Input: part model. Units: mm. Frame: model coordinates. Round coordinates to 2 decimals unless told otherwise and drop trailing zeros. Loops run counter-clockwise (first coordinate to the right, second up) from the corner with the lowest first, then second, coordinate; pieces in that order, holes last. Notation, with made-up numbers: (27, 58.5) -> (71, 58.5) arc R23 ccw to (71, 70.5) -> close; hole circle Ø9 at (87, 70). An arc over 180 degrees is marked (long way). Answer as a JSON object with one key per item and string values. Group by question number.
Item 1: Section query A-A on x = -4. Return loops of the section in (y, z).
Item 2: Section query B-B on x = 132.5. Return loops of the section in (y, z), and give its area (3 significant figures).
Item 3: Material intervals for line 1 (Z direction, x = -11.5, y = 0); line 2 (Y direction, x = -7, z = 3); line 3 (Z direction, x = -16.5, y = -3.5), sorted ascending. Write a range as [from, to].
Item 4: Draft query along Z for faces 1 (the cylindrical face through (-14.255, -2.979, -13.413)), 2 (the flat face through (-26.778, 9, -11)), 3 (the conical face through (106.719, 4.046, 6.346)), 4 (the conical face through (98.54, -1.59, -7.18)). Return one class per face: released by +Z, released by -Z, zero draft, split by the parting line, or undercut.
Item 5: Pin query (flat end, axial travel): pin 1 (8 mm diameter, centred on x = 181, z = -1.5, fed in from -Y); pin 2 (2 mm diameter, centred on x = 166.5, y = 1.5, fed in from +Z); pin 3 (1.5 mm diameter, centred on x = 61, y = 1, fed in from +Z). Return the tip coordinate at first contact, or that it passes through.
from build123d import *


with BuildPart() as part:
    # Sketch1 → Revolve1 (revolve)
    with BuildSketch(Plane.XY):
        with BuildLine():
            Line((-26.777640385, 14.5), (-1.377640385, 14.5))
            ThreePointArc((-1.377640385, 14.5), (-1.305458082, 14.529361179), (-1.274265968, 14.600771373))
            ThreePointArc((-1.274265968, 14.600771373), (-1.050186045, 15.089583285), (-0.541877208, 15.265))
            Line((-0.541877208, 15.265), (211.018122792, 0))
            Line((211.018122792, 0), (200.457781941, 0))
            Line((200.457781941, 0), (-0.569260312, 14.505))
            ThreePointArc((-0.569260312, 14.505), (-0.603115726, 14.493556272), (-0.618623339, 14.461359037))
            ThreePointArc((-0.618623339, 14.461359037), (-0.854079086, 13.949106575), (-1.377640385, 13.74))
            Line((-1.377640385, 13.74), (-26.777640385, 13.74))
            Line((-26.777640385, 13.74), (-26.777640385, 14.5))
        make_face()
    revolve(axis=Axis((0, 0, 0), (1, 0, 0)))


solid = part.part
Solved:
{
 "1": {"outline": "circle Ø29 at (0, 0); hole circle Ø27.48 at (0, 0)"},
 "2": {"outline": "circle Ø11.33 at (0, 0); hole circle Ø9.81 at (0, 0)", "area": "25.3 mm²"},
 "3": {"line 1": "[-14.5, -13.74], [13.74, 14.5]", "line 2": "[-14.19, -13.41], [13.41, 14.19]", "line 3": "[-14.07, -13.29], [13.29, 14.07]"},
 "4": {"face 1": "undercut", "face 2": "zero draft", "face 3": "split by the parting line", "face 4": "undercut"},
 "5": {"pin 1": "y = -2.43", "pin 2": "z = 3.19", "pin 3": "z = 10.85"}
}
